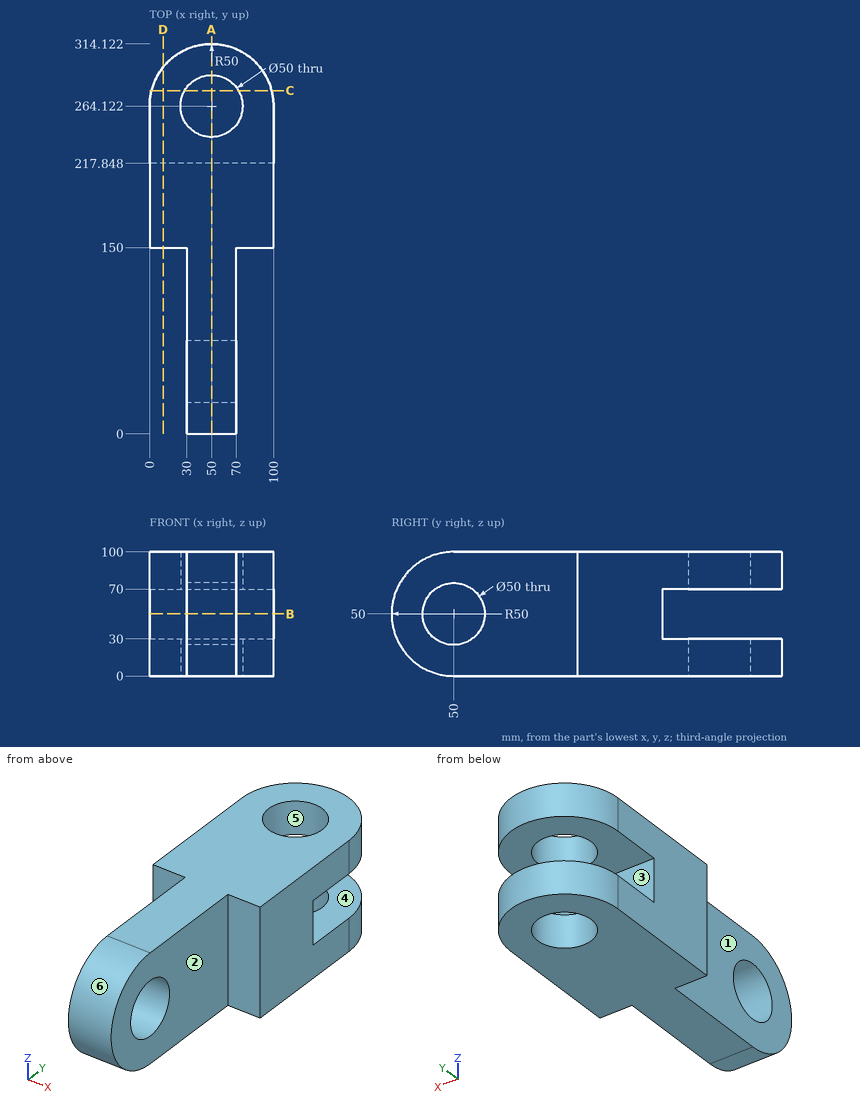
The drawing under review shows one solid part. Ordinate dimensions are in mm from its lowest x, y, z. A direction names the side the tool comes from. Round coordinates to 2 decimals unless told otherwise and drop trailing zeros. Write each loop counter-clockwise with the first axis right and the second up, starting at its lowest first coordinate (ties: lowest second). Pieces come first, ordered by that corner, then holes.
(1) Mouldability with a two-part tool opening along Y and no side actions: class the marked faces 4, 5 and 6 as +Y half, -Y half, draft (parallel to the pull), parting line (faces both ways), or undercut.
(2) We need section B-B on z = 50. Give the boundary of the cut face in (x, y), and give its area (3 significant figures).
(3) Insertion check: pin 1 (10 mm diameter, centred on x = 46.5, z = 68.5, fed in from -Y); pin 2 (8 mm diameter, centred on x = 61, z = 84, fed in from -Y); pin 3 (2 mm diameter, centred on x = 14.5, z = 77.5, fed in from -Y); pin 4 (3 mm diameter, centred on x = 27, y = 101, fed in from +Z). Each pin has a flat end and moves straight along its axis. Give the tip position at first contact, or say it passes through.
(4) We need section C-C on y = 276.5. Give the boundary of the cut face in (x, z).
(5) We need section D-D on x = 11. Give the boundary of the cut face in (y, z), and give its area (3 significant figures).
(6) Machinability: for the marked faces 1, 2 and 3, which of the approach directions +Z, -Z, +X, -X, +Y, -Y give a long, thin tool a straight path to every point of the face, cutting with its end or side? Answer none if there is none.
(7) Wall thickness on L1, parallel to Y at x = 45, z = 50; L2, parallel to Z at x = 85.5, y = 282.5; L3, parallel to Y at x = 79, z = 58: over which ranges is each line inside the solid? List them lowest first.
(8) We need section A-A on x = 50. Give the boundary of the cut face in (y, z), and give its area (3 significant figures).
Findings below:
1. face 4: draft
1. face 5: undercut
1. face 6: -Y half
2. outline: (0, 150) - (30, 150) - (30, 75) - (70, 75) - (70, 150) - (100, 150) - (100, 217.85) - (0, 217.85) - close; (30, 0) - (70, 0) - (70, 25) - (30, 25) - close
2. area: 10,800 mm2
3. pin 1: stops at y = 1.86
3. pin 2: stops at y = 10
3. pin 3: stops at y = 150
3. pin 4: passes through
4. outline: (1.56, 0) - (28.28, 0) - (28.28, 30) - (1.56, 30) - close; (1.56, 70) - (28.28, 70) - (28.28, 100) - (1.56, 100) - close; (71.72, 0) - (98.44, 0) - (98.44, 30) - (71.72, 30) - close; (71.72, 70) - (98.44, 70) - (98.44, 100) - (71.72, 100) - close
5. outline: (150, 0) - (295.41, 0) - (295.41, 30) - (217.85, 30) - (217.85, 70) - (295.41, 70) - (295.41, 100) - (150, 100) - close
5. area: 11,400 mm2
6. face 1: +Z, -Z, -X, -Y
6. face 2: +Z, -Z, +X, -Y
6. face 3: +X, -X, +Y
7. L1: y = 0 to 25, 75 to 217.85
7. L2: z = 0 to 30, 70 to 100
7. L3: y = 150 to 217.85
8. outline: (50, 0) - (239.12, 0) - (239.12, 30) - (217.85, 30) - (217.85, 70) - (239.12, 70) - (239.12, 100) - (50, 100) arc R50 ccw to start; (289.12, 0) - (314.12, 0) - (314.12, 30) - (289.12, 30) - close; (289.12, 70) - (314.12, 70) - (314.12, 100) - (289.12, 100) - close; hole circle Ø50 at (50, 50)
8. area: 21,500 mm2
